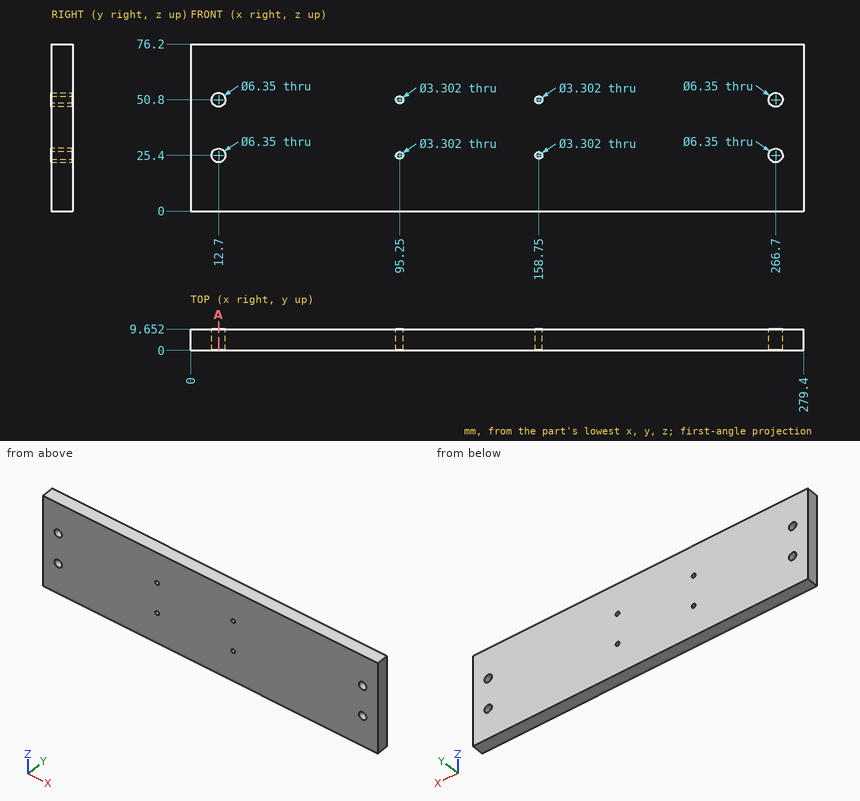
Verification items for this drawing (mm, ordinates from the low corner). Round coordinates to 2 decimals unless told otherwise and drop trailing zeros. Write each loop counter-clockwise with the first axis right and the second up, starting at its lowest first coordinate (ties: lowest second). Pieces come first, ordered by that corner, then holes. Notation, with made-up numbers: M 53.25,29 L 57.25,29 A16 ccw 57.25,46 Z; hole C 84,10.5 d5. An arc over 180 degrees is marked long. Write item = value, one per line. Start each with the question number.
1. Section check A-A, the plane x = 12.7. Record the cut outline in (y, z) (3 decimals).
2. Scan lines: line 1 (X direction, y = 7.25, z = 25.4) (3 decimals); line 2 (Z direction, x = 95.25, y = 3.25); line 3 (Z direction, x = 266.7, y = 6.75) (3 decimals). Record each from-to range of solid material in increasing order. Write a range as [from, to].
3. Gauge pin test, flat end, axial feed: pin 1 (3 mm diameter, centred on x = 158.75, z = 50.8, fed in from -Y). Record the tip position at first contact, or that the pin passes through.
Results found:
q1.outline = M 0,0 L 9.652,0 L 9.652,22.225 L 0,22.225 Z; M 0,28.575 L 9.652,28.575 L 9.652,47.625 L 0,47.625 Z; M 0,53.975 L 9.652,53.975 L 9.652,76.2 L 0,76.2 Z
q2.line_1 = [0, 9.525], [15.875, 93.599], [96.901, 157.099], [160.401, 263.525], [269.875, 279.4]
q2.line_2 = [0, 23.75], [27.05, 49.15], [52.45, 76.2]
q2.line_3 = [0, 22.225], [28.575, 47.625], [53.975, 76.2]
q3.pin_1 = through
